Autodesk Inventor part; units mm, degrees
ref_plane "YZ Plane" through (0, 0, 0) normal (1, 0, 0) x (0, 1, 0)
ref_plane "XZ Plane" through (0, 0, 0) normal (0, 1, 0) x (-1, 0, 0)
ref_plane "XY Plane" through (0, 0, 0) normal (0, 0, 1) x (1, 0, 0)
sketch "Sketch1" plane through (0, 0, 0) normal (0, 1, 0) x (-1, 0, 0)
  line L0 (0, 0) -> (67.31, 0)
  line L1 (67.31, 0) -> (67.31, -40.005)
  line L2 (67.31, -40.005) -> (0, -40.005)
  line L3 (0, -40.005) -> (0, 0)
  dimension "d0" = 40.005
  dimension "d1" = 67.31
extrude "Extrusion1" add sketch "Sketch1" along normal blind 3.175
sketch "Sketch2" plane through (0, 3.175, 0) normal (0, 1, 0) x (1, 0, 0)
  circle A0 centre (-13.97, 27.305) radius 4.445
  line L0 (0, 0) -> (0, 40.005)
  line L1 (-67.31, 0) -> (0, 0)
  line L2 (0, 40.005) -> (-67.31, 40.005)
  circle A1 centre (-5.08, 6.35) radius 1.5875
  circle A2 centre (-22.68, 6.35) radius 1.5875
  dimension "d4" = 13.97
  dimension "d28" = 12.7
  dimension "d29" = 8.89
  dimension "d30" = 3.175
  dimension "d31" = 3.175
  dimension "d32" = 5.08
  dimension "d33" = 17.6
  dimension "d34" = 6.35
  dimension "d35" = 6.35
extrude "Extrusion2" cut sketch "Sketch2" against normal blind 6.35
sketch "Sketch3" plane through (0, 0, 0) normal (0, -1, 0) x (1, 0, 0)
  line L0 (0, -40.005) -> (-67.31, -40.005)
  line L1 (-67.31, 0) -> (0, 0)
  line L2 (-67.31, -40.005) -> (-35.56, -40.005)
  line L3 (-35.56, -40.005) -> (-35.56, 0)
  line L4 (-35.56, 0) -> (-67.31, 0)
  line L5 (-67.31, 0) -> (-67.31, -40.005)
  point P0 (-67.31, 0)
  point P1 (-35.56, -40.005)
  dimension "d8" = 31.75
extrude "Extrusion3" add sketch "Sketch3" along normal blind 19.05
sketch "Sketch6" plane through (0, 3.175, 0) normal (0, 1, 0) x (1, 0, 0)
  circle A0 centre (-55.88, 28.575) radius 2.1828
  circle A1 centre (-55.88, 9.525) radius 2.1828
  line L0 (-67.31, 40.005) -> (-67.31, 0)
  line L1 (-67.31, 0) -> (0, 0)
  dimension "d19" = 4.3656
  dimension "d20" = 4.3656
  dimension "d21" = 11.43
  dimension "d22" = 11.43
  dimension "d23" = 19.05
  dimension "d24" = 9.525
extrude "Extrusion6" cut sketch "Sketch6" against normal blind 25.4
fillet "Fillet1" radius 1.27 9 edges at (0, 0, -20.0025) (-17.78, 0, 0) (-17.78, 0, -40.005) (-35.56, -9.525, 0) (0, 1.5875, 0) (0, 1.5875, -40.005) (-67.31, -7.9375, -40.005) (-35.56, -9.525, -40.005) (-67.31, -7.9375, 0)
sketch "Sketch7" plane through (0, 0, 0) normal (0, -1, 0) x (1, 0, 0)
  circle A0 centre (-13.97, -15.24) radius 3.175
  line L0 (-1.27, 0) -> (-36.83, 0)
  line L1 (0, -38.735) -> (0, -1.27)
  point P0 (0, 0)
  dimension "d36" = 6.35
  dimension "d37" = 15.24
  dimension "d38" = 13.97
extrude "Extrusion7" cut sketch "Sketch7" against normal blind 2.54
properties part number "SwerveDriveBracket_C"
Read the model definition and answer for the solid it produces. Units are mm, in the model's axes. A direction names the side the tool comes from. Coordinates: 2 decimals unless noted, no trailing zeros. Write each loop counter-clockwise with the first axis right and the second up, starting at its lowest first coordinate (ties: lowest second). Pieces come first, ordered by that corner, then holes. Notation, with made-up numbers: (85.5, -2.75) -> (122.5, -2.75) arc R35 cw to (122.5, 35.25) -> close; hole circle Ø6 at (39.5, 80.5). An arc over 180 degrees is marked (long way). Write item = value, one per line.
(1) Section C-C on x = -55.88 is taken. Write down the section's boundary in (y, z) (3 decimals).
From the geometry:
outline = (-19.05, -40.005) -> (3.175, -40.005) -> (3.175, -30.758) -> (-19.05, -30.758) -> close; (-19.05, -26.392) -> (3.175, -26.392) -> (3.175, -11.708) -> (-19.05, -11.708) -> close; (-19.05, -7.342) -> (3.175, -7.342) -> (3.175, 0) -> (-19.05, 0) -> close
(2) Section B-B on x = -22.68 is taken. Write down the section's boundary in (y, z) (1 decimal).
From the geometry:
outline = (0, -38.7) arc R1.3 ccw to (1.3, -40) -> (3.2, -40) -> (3.2, -7.9) -> (0, -7.9) -> close; (0, -4.8) -> (3.2, -4.8) -> (3.2, 0) -> (1.3, 0) arc R1.3 ccw to (0, -1.3) -> close
(3) Given pin 1 Ø4 at (x, z) = (-22.68, -6.35) entering from -Y; pin 2 Ø3 at (y, z) = (-11.5, -22.5) entering from +X; pin 3 Ø3 at (x, y) = (-30.5, -0.5) entering from +Z, each flat-ended and moving along its own axis, determine where each tip first touches the part or whether it passes through.
From the geometry:
pin_1 = 0
pin_2 = -35.56
pin_3 = -0.03
(4) For a pull along Z with two mould halves and no side action, classify faces 4 (the face through (-0.36, 2.24, -39.62)), 5 (the face through (-14.934, 1.61, -22.966)), 6 (the face through (-0.382, 0.362, -19.74)) as +Z half, -Z half, draft (parallel to the pull), parting line (faces both ways), or undercut.
From the geometry:
face_4 = -Z half
face_5 = undercut
face_6 = draft
(5) Which of the six approach directions +Z, -Z, +X, -X, +Y, -Y give full straight-line access (tool end or side, diameter ignored) to faces 1 (the face through (-35.922, -9.032, -0.382)), 2 (the face through (-35.56, -9, -20)), 3 (the face through (-12.263, 1.252, -12.563))?
From the geometry:
face_1 = +Z, +X, -Y
face_2 = +Z, -Z, +X, -Y
face_3 = -Y
(6) Straight lines are drawn through the part: L1, parallel to Z at x = -13.97, y = 1.3 (3 decimals); L2, parallel to Z at x = -55.88, y = -11 (3 decimals); L3, parallel to X at y = 2.4, z = -6.35. For each, find the intervals that lie inside material, in ascending order. Write a range as from..to.
From the geometry:
L1 = -40.005..-31.75, -22.86..-18.415, -12.065..0
L2 = -40.005..-30.758, -26.392..-11.708, -7.342..0
L3 = -67.31..-24.27, -21.09..-6.67, -3.49..0
(7) Section D-D on z = -20.5 is taken. Write down the section's boundary in (x, y) (3 decimals).
From the geometry:
outline = (-67.31, -19.05) -> (-35.56, -19.05) -> (-35.56, 0) -> (-1.27, 0) arc R1.27 ccw to (0, 1.27) -> (0, 3.175) -> (-67.31, 3.175) -> close
(8) Section A-A on z = -6.35 is taken. Count the separate pieces of the cut face and the enclosed holes in it, plus the area to 3 significant figures.
From the geometry:
separate_pieces = 3
enclosed_holes = 0
area = 798 mm2
